Input: part model. Units: mm. Frame: model coordinates. A direction names the side the tool comes from. Coordinates: 2 decimals unless noted, no trailing zeros. Order: outer loops, then holes, each group sorted by start corner. A loop starts at its lowest first (then second) coordinate and runs counter-clockwise, first axis right, second up.
from build123d import *

# Parameters (mm, degrees)
SKETCH1_R                = 25.969085179
BOSS_EXTRUDE1_DEPTH      = 10
CUT_EXTRUDE6_DEPTH       = 10
CUT_EXTRUDE6_DEPTH_BACK  = 10
SKETCH2_R                = 6.5
SKETCH4_R                = 5.101859566
BOSS_EXTRUDE2_DEPTH      = 50
BOSS_EXTRUDE3_DEPTH      = 1
BOSS_EXTRUDE3_DEPTH_BACK = 5
SKETCH5_R                = 27.403110043
SKETCH6_R                = 3.156893789
CUT_EXTRUDE7_DEPTH       = 6
CIRPATTERN1_COUNT        = 4


with BuildPart() as part:
    # Sketch1 → Boss-Extrude1 (new body)
    with BuildSketch(Plane(origin=(0, 0, 0), x_dir=(1, 0, 0), z_dir=(0, 1, 0))):
        with Locations(Location((0, 0, 0), (0, 0, 270))):
            Circle(SKETCH1_R)
    extrude(amount=BOSS_EXTRUDE1_DEPTH)

    # Sketch2 → Cut-Extrude6 (cut, two sides: drawn at the far end of the back side and taken through both)
    with BuildSketch(Plane(origin=(0, 0, 0), x_dir=(1, 0, 0), z_dir=(0, 1, 0)).offset(-CUT_EXTRUDE6_DEPTH_BACK)):
        with Locations(Location((-10.19719706, 11.000780524, 0), (0, 0, 270))):
            Circle(SKETCH2_R)
        with Locations(Location((-11.032390275, -10.162989955, 0), (0, 0, 270))):
            Circle(SKETCH2_R)
        with Locations(Location((10.330398744, -10.875792467, 0), (0, 0, 270))):
            Circle(SKETCH2_R)
        with Locations(Location((9.448943305, 11.649784136, 0), (0, 0, 270))):
            Circle(SKETCH2_R)
    extrude(amount=CUT_EXTRUDE6_DEPTH + CUT_EXTRUDE6_DEPTH_BACK, mode=Mode.SUBTRACT)

    # Sketch4 → Boss-Extrude2 (add)
    with BuildSketch(Plane(origin=(0, 0, 0), x_dir=(1, 0, 0), z_dir=(0, 1, 0))):
        with Locations(Location((-20.316325534, 19.065240611, 0), (0, 0, 20.088676174))):
            Circle(SKETCH4_R)
        with Locations(Location((19.683674466, 19.065240611, 0), (0, 0, 155.604859665))):
            Circle(SKETCH4_R)
    boss_extrude2 = extrude(amount=BOSS_EXTRUDE2_DEPTH)

    # Mirror1: Boss-Extrude2 across plane
    add(boss_extrude2.mirror(Plane.XY))

    # Sketch5 → Boss-Extrude3 (add, two sides: drawn at the far end of the back side and taken through both)
    with BuildSketch(Plane(origin=(0, 50, 0), x_dir=(1, 0, 0), z_dir=(0, 1, 0)).offset(-BOSS_EXTRUDE3_DEPTH_BACK)):
        with Locations(Location((0, 0, 0), (0, 0, 270))):
            Circle(SKETCH5_R)
    extrude(amount=BOSS_EXTRUDE3_DEPTH + BOSS_EXTRUDE3_DEPTH_BACK)

    # Sketch6 → Cut-Extrude7 (cut)
    with BuildSketch(Plane(origin=(0, 51, 0), x_dir=(1, 0, 0), z_dir=(0, 1, 0))):
        with Locations(Location((8, 8, 0), (0, 0, 270))):
            Circle(SKETCH6_R)
    cut_extrude7 = extrude(amount=-CUT_EXTRUDE7_DEPTH, mode=Mode.SUBTRACT)

    # CirPattern1: Cut-Extrude7 ×4 about axis
    cirpattern1_axis = Axis((-0.107600069, 0, 0.107600069), (0, 1, 0))
    for i in range(1, CIRPATTERN1_COUNT):
        add(cut_extrude7.rotate(cirpattern1_axis, i * 360 / CIRPATTERN1_COUNT), mode=Mode.SUBTRACT)


solid = part.part
Item 1: Ray query, probe 1 along Y at (x, z) = (15, 3); probe 2 along Z at (x, y) = (-6.5, 8.5); probe 3 along Y at (x, z) = (23, 22). Return the intervals inside material, ascending.
Response values:
probe 1: y = 0 to 10, 45 to 51
probe 2: z = -25.14 to -16.35, -5.65 to 5.5, 14.82 to 25.14
probe 3: y = 0 to 50
Item 2: Access query for faces 5 (the face through (22, 50, -21)), 6 (the face through (-22, 50, -20)), 7 (the face through (11.4, 4.93, -5.45)), 8 (the face through (-22.678, 24.65, -23.588)). Directions: +Z, -Z, +X, -X, +Y, -Y. A direction counts if a zero-diameter tool reaches every point of the face in a straight line with its end or side. Return the directions, or none.
Response values:
face 5: -Z, +X, +Y
face 6: -Z, -X, +Y
face 7: -Y
face 8: none
Item 3: Pin query (flat end, axial travel): pin 1 Ø1.5 at (x, y) = (13, 43.5) entering from -Z; pin 2 Ø4.5 at (x, z) = (-23, -19) entering from +Y; pin 3 Ø6 at (x, y) = (12, 9) entering from +Z; pin 4 Ø1.5 at (y, z) = (37, 16.5) entering from +X. Return the tip coordinate at first contact, or that it passes through.
Response values:
pin 1: passes through
pin 2: stops at y = 50
pin 3: stops at z = 24.36
pin 4: stops at x = 24.45
Item 4: Cut plane A-A on x = 0. Return loops of the section in (y, z).
Response values:
outline: (0, -25.97) - (10, -25.97) - (10, 25.97) - (0, 25.97) - close; (45, -27.4) - (51, -27.4) - (51, 27.4) - (45, 27.4) - close
Item 5: Cut plane B-B on z = 0. Return loops of the section in (x, y), then the cut area to 3 significant figures.
Response values:
outline: (-27.4, 45) - (27.4, 45) - (27.4, 51) - (-27.4, 51) - close; (-25.97, 0) - (25.97, 0) - (25.97, 10) - (-25.97, 10) - close
area: 848 mm2
Item 6: Draft query along X for faces 1 (the face through (-10.75, 4.93, 3.67)), 2 (the face through (25.97, 4.93, 0.21)), 3 (the face through (0, 51, 0)), 4 (the face through (0, 10, 0)). Return one class per face: pulls with the +X half, pulls with the -X half, needs draft (parallel to the pull), parting line crosses it, or undercut.
Response values:
face 1: undercut
face 2: pulls with the +X half
face 3: needs draft
face 4: undercut
Item 7: Cut plane C-C on z = -8. Return loops of the section in (x, y).
Response values:
outline: (-26.21, 45) - (-11.37, 45) - (-11.37, 51) - (-26.21, 51) - close; (-24.71, 0) - (-15.96, 0) - (-15.96, 10) - (-24.71, 10) - close; (-5.06, 45) - (4.84, 45) - (4.84, 51) - (-5.06, 51) - close; (-4.43, 0) - (4.07, 0) - (4.07, 10) - (-4.43, 10) - close; (11.16, 45) - (26.21, 45) - (26.21, 51) - (11.16, 51) - close; (14.83, 0) - (24.71, 0) - (24.71, 10) - (14.83, 10) - close
Item 8: Cut plane D-D on x = 6. Return loops of the section in (y, z).
Response values:
outline: (0, -25.27) - (10, -25.27) - (10, -17.16) - (0, -17.16) - close; (0, -6.14) - (10, -6.14) - (10, 6.03) - (0, 6.03) - close; (0, 15.72) - (10, 15.72) - (10, 25.27) - (0, 25.27) - close; (45, -26.74) - (51, -26.74) - (51, -10.44) - (45, -10.44) - close; (45, -5.56) - (51, -5.56) - (51, 5.77) - (45, 5.77) - close; (45, 10.66) - (51, 10.66) - (51, 26.74) - (45, 26.74) - close
